```python
from build123d import *

# Parameters (mm, degrees)
F1_DEPTH = 90
F2_W     = 29.6450741589
F2_H     = 70.9077940881
F3_DEPTH = 25


with BuildPart() as f1:
    # F0 (on Front) → F1 (new body)
    with BuildSketch(Plane.XZ):
        with BuildLine():
            Line((19.7393086681, -2.1245502867), (12.1618005228, -2.1245502867))
            ThreePointArc((12.1618005228, -2.1245502867), (-3.2044417421, -13.8565980652), (-10.4731612691, 4.0578671196))
            Line((-10.4731612691, 4.0578671196), (-17.5973851442, 6.8181754041))
            ThreePointArc((-17.5973851442, 6.8181754041), (-4.5978304439, -21.3209109289), (19.7393086681, -2.1245502867))
        make_face()
        with BuildLine():
            ThreePointArc((-17.5973851442, 6.8181754041), (4.5978304439, 17.0718103555), (19.7393086681, -2.1245502867))
            Line((19.7393086681, -2.1245502867), (47.8034389698, -2.1245502867))
            ThreePointArc((47.8034389698, -2.1245502867), (56.8842174331, 15.549580718), (76.5405482344, 18.4588939876))
            Line((76.5405482344, 18.4588939876), (72.7407261729, 29.9625266343))
            Line((72.7407261729, 29.9625266343), (84.2738300562, 53.3970333636))
            Line((84.2738300562, 53.3970333636), (71.2432563305, 47.4482923746))
            Line((71.2432563305, 47.4482923746), (15.4384011403, 50.5643002689))
            Line((15.4384011403, 50.5643002689), (-38.3835434914, 14.8718534037))
            Line((-38.3835434914, 14.8718534037), (-17.5973851442, 6.8181754041))
        make_face()
        with BuildLine():
            Line((57.3760422717, -2.1245502867), (47.8034389698, -2.1245502867))
            ThreePointArc((47.8034389698, -2.1245502867), (69.5436149836, -23.8647263004), (91.2837909973, -2.1245502867))
            ThreePointArc((91.2837909973, -2.1245502867), (87.2177459882, 10.5348472637), (76.5405482344, 18.4588939876))
            Line((76.5405482344, 18.4588939876), (76.9786015153, 17.1327255666))
            Line((76.9786015153, 17.1327255666), (73.9260684349, 9.2263936144))
            ThreePointArc((73.9260684349, 9.2263936144), (79.5778973875, 4.7575280576), (81.7111876954, -2.1245502867))
            ThreePointArc((81.7111876954, -2.1245502867), (69.5436149836, -14.2921229985), (57.3760422717, -2.1245502867))
        make_face()
        with BuildLine():
            ThreePointArc((-10.4731612691, 4.0578671196), (3.2044417421, 9.6074974918), (12.1618005228, -2.1245502867))
            Line((12.1618005228, -2.1245502867), (19.7393086681, -2.1245502867))
            ThreePointArc((19.7393086681, -2.1245502867), (4.5978304439, 17.0718103555), (-17.5973851442, 6.8181754041))
            Line((-17.5973851442, 6.8181754041), (-10.4731612691, 4.0578671196))
        make_face()
        with BuildLine():
            ThreePointArc((76.5405482344, 18.4588939876), (56.8842174331, 15.549580718), (47.8034389698, -2.1245502867))
            Line((47.8034389698, -2.1245502867), (57.3760422717, -2.1245502867))
            ThreePointArc((57.3760422717, -2.1245502867), (62.6615366393, 7.9097321173), (73.9260684349, 9.2263936144))
            Line((73.9260684349, 9.2263936144), (76.9786015153, 17.1327255666))
            Line((76.9786015153, 17.1327255666), (76.5405482344, 18.4588939876))
        make_face()
    extrude(amount=F1_DEPTH)

    # F2 (on face) → F3 (cut)
    with BuildSketch(Plane(origin=(-18.5741359404, 0, 28.0086181803), x_dir=(0.8333974675, 0, 0.5526741003), z_dir=(-0.5526741003, 0, 0.8333974675))):
        with Locations((16.7337115854, -45)):
            Rectangle(F2_W, F2_H)
    extrude(amount=-F3_DEPTH, mode=Mode.SUBTRACT)


solid = f1.part
```
Work out the finished part from the listing and answer in its coordinate system (mm). A direction names the side the tool comes from. Round coordinates to 2 decimals unless told otherwise and drop trailing zeros. Write each loop counter-clockwise with the first axis right and the second up, starting at its lowest first coordinate (ties: lowest second). Pieces come first, ordered by that corner, then holes. Notation, with made-up numbers: (-35, 36.5) - (-19, 36.5) arc R16 ccw to (-19, 62.5) - close; hole circle Ø8 at (52, 15). An arc over 180 degrees is marked (long way). Return JSON: item names as keys, results as strings. Group by question number.
Q1. Find the intervals of material crossed by L1, parallel to Y at x = -1.5, z = 15; L2, parallel to X at y = -34, z = -13; L3, parallel to Z at x = 63.5, y = -8, in increasing order.
Q2. The mould has two halves that part along X. Classify faces 5 (the flat face through (26, -90, 15)), 6 (the flat face through (2, -80.454, 27)), 7 (the flat face through (78.43, -44.37, 41.52)): released by +X, released by -X, zero draft, split by the parting line, or undercut.
Q3. The part is cut by section B-B on x = 1.5. Write down the section's boundary in (y, z).
Q4. Each of these flat-tipped pins is pushed along its axis until it touches: pin 1 Ø5 at (x, y) = (-23, -31.5) entering from +Z; pin 2 Ø5 at (x, y) = (48, -41.5) entering from -Z; pin 3 Ø10 at (x, y) = (53, -76) entering from -Z. Where does it stop, or does it pass through?
Q5. The part is cut by section A-A on y = -52. Write down the section's boundary in (x, z), then the cut area to 3 significant figures.
Q6. The part is cut by section C-C on z = 43.5. Write down the section's boundary in (x, y), then the cut area to 3 significant figures.
Q7. The part is cut by section D-D on x = -28. Write down the section's boundary in (y, z), then the cut area to 3 significant figures.
Q8. For faces 1 (the flat face through (34, -44, -2.125)), 2 (the flat face through (74.667, -44.37, 24.13)), 3 (the flat face through (43.731, -44.37, 48.984)), 4 (the flat face through (14.536, -45.496, 35.177)), determine the directions among +Z, -Z, +X, -X, +Y, -Y from which every point of the face is accessible in a straight line to the end or side of a thin tool.
Solved:
{
 "1": {"L1": "-90 to -80.45, -9.55 to 0", "L2": "-16.47 to -5.44, 5.44 to 16.47, 50.72 to 64.09, 75 to 88.37", "L3": "-23.01 to -12.69, 8.44 to 47.88"},
 "2": {"face 5": "zero draft", "face 6": "undercut", "face 7": "released by +X"},
 "3": {"outline": "(-90, -21.81) - (0, -21.81) - (0, -14.19) - (-90, -14.19) - close; (-90, 9.94) - (0, 9.94) - (0, 41.32) - (-9.55, 41.32) - (-9.55, 11.32) - (-80.45, 11.32) - (-80.45, 41.32) - (-90, 41.32) - close"},
 "4": {"pin 1": "z = 26.73", "pin 2": "z = -12.61", "pin 3": "z = -20.55"},
 "5": {"outline": "(-38.38, 14.87) - (-17.6, 6.82) arc R19.74 ccw (long way) to (19.74, -2.12) - (47.8, -2.12) arc R21.74 ccw (long way) to (76.54, 18.46) - (72.74, 29.96) - (84.27, 53.4) - (71.24, 47.45) - (15.44, 50.56) - (7.72, 45.45) - (21.54, 24.61) - (-0.45, 10.03) arc R12.16 cw (long way) to (-3.93, 9.38) - (-16.98, 29.06) - close; hole circle Ø24.34 at (69.54, -2.12)", "area": "4,660 mm²"},
 "6": {"outline": "(4.79, -90) - (79.4, -90) - (79.4, 0) - (4.79, 0) - (4.79, -9.55) - (9.02, -9.55) - (9.02, -80.45) - (4.79, -80.45) - close", "area": "6,420 mm²"},
 "7": {"outline": "(-90, 10.85) - (0, 10.85) - (0, 21.76) - (-90, 21.76) - close", "area": "982 mm²"},
 "8": {"face 1": "-Z, +Y, -Y", "face 2": "+X, +Y, -Y", "face 3": "+Z, +Y, -Y", "face 4": "none"}
}
